Read the model definition and answer for the solid it produces. Units are mm, in the model's axes. A direction names the side the tool comes from. Round coordinates to 2 decimals unless told otherwise and drop trailing zeros. Order: outer loops, then holes, each group sorted by start corner. A loop starts at its lowest first (then second) coordinate and runs counter-clockwise, first axis right, second up.
from build123d import *

# Parameters (mm, degrees)
SKETCH1_R           = 2.286
BOSS_EXTRUDE1_DEPTH = 7.9375
SKETCH2_R           = 2.286
CUT_EXTRUDE1_DEPTH  = 13.335
CUT_EXTRUDE2_START  = 0.79375
CUT_EXTRUDE2_DEPTH  = 2.794
CHAMFER1_SIZE       = 1.5875


with BuildPart() as part:
    # Sketch1 → Boss-Extrude1 (new body)
    with BuildSketch(Plane.XY):
        with BuildLine():
            Line((-5.55625, 4.7625), (-5.55625, 18.0975))
            Line((-5.55625, 18.0975), (5.55625, 18.0975))
            Line((5.55625, 18.0975), (5.55625, 4.7625))
            Line((5.55625, 4.7625), (4.706470588, -0.728382353))
            ThreePointArc((4.706470588, -0.728382353), (0, -4.7625), (-4.706470588, -0.728382353))
            Line((-4.706470588, -0.728382353), (-5.55625, 4.7625))
        make_face()
        with Locations(Location((0, 0, 0), (0, 0, 270))):
            Circle(SKETCH1_R, mode=Mode.SUBTRACT)
    extrude(amount=BOSS_EXTRUDE1_DEPTH)

    # Sketch2 → Cut-Extrude1 (cut)
    with BuildSketch(Plane(origin=(0, 18.0975, 0), x_dir=(1, 0, 0), z_dir=(0, 1, 0))):
        with Locations(Location((2.54e-07, -4.318750409, 0), (0, 0, 270))):
            Circle(SKETCH2_R)
    extrude(amount=-CUT_EXTRUDE1_DEPTH, mode=Mode.SUBTRACT)

    # Sketch3 → Cut-Extrude2 (cut)
    with BuildSketch(Plane(origin=(0, 4.7625, 0), x_dir=(1, 0, 0), z_dir=(0, 1, 0)).offset(CUT_EXTRUDE2_START)):
        Polygon((-1.906410334, -1.016750409), (-4.156524955, -4.914063255), (-4.156524955, -7.9375), (4.156521786, -7.9375), (4.156521786, -4.914056884), (1.906410843, -1.016750409), align=None)
    extrude(amount=CUT_EXTRUDE2_DEPTH, mode=Mode.SUBTRACT)

    # Chamfer1
    chamfer1_edges = [part.edges().sort_by_distance(p)[0] for p in [
        (-5.55625, 18.0975, 3.96875),
        (5.55625, 18.0975, 3.96875),
    ]]
    chamfer(chamfer1_edges, length=CHAMFER1_SIZE)


solid = part.part
Q1. A cutting plane is placed at B-B, the plane y = 8.75. Give the vertices of the cut face in (x, z).
Outcome:
outline: (-5.56, 0) - (5.56, 0) - (5.56, 7.94) - (-5.56, 7.94) - close; hole circle Ø4.57 at (0, 4.32)
Q2. A cutting plane is placed at D-D, the plane y = 0. Give the vertices of the cut face in (x, z), plus the area to 3 significant figures.
Outcome:
outline: (-4.82, 0) - (-2.29, 0) - (-2.29, 7.94) - (-4.82, 7.94) - close; (2.29, 0) - (4.82, 0) - (4.82, 7.94) - (2.29, 7.94) - close
area: 40.2 mm2
Q3. Flat-ended cylindrical pins translate along their axes: pin 1 (4 mm diameter, centred on x = 0, z = 4.32, fed in from +Y); pin 2 (2 mm diameter, centred on x = 1, y = 7, fed in from +Z). Find the tip coordinate at first contact, or state that the pin passes through.
Outcome:
pin 1: stops at y = 4.76
pin 2: stops at z = 1.18
Q4. Straight lines are drawn through the part: probe 1 along X at (y, z) = (10.5, 4.25); probe 2 along Y at (x, z) = (-1.5, 2); probe 3 along X at (y, z) = (6.75, 5.75). For each, find the intervals that lie inside material, in ascending order.
Outcome:
probe 1: x = -5.56 to -2.28, 2.28 to 5.56
probe 2: y = -4.52 to -1.73, 1.73 to 5.56, 8.35 to 18.1
probe 3: x = -5.56 to -4.16, 4.16 to 5.56
Q5. A cutting plane is placed at C-C, the plane z = 5.75. Give the vertices of the cut face in (x, y) (1 decimal).
Outcome:
outline: (-5.6, 4.8) - (-4.7, -0.7) arc R4.8 ccw to (4.7, -0.7) - (5.6, 4.8) - (5.6, 16.5) - (4, 18.1) - (1.8, 18.1) - (1.8, 8.4) - (4.2, 8.4) - (4.2, 5.6) - (1.8, 5.6) - (1.8, 4.8) - (-1.8, 4.8) - (-1.8, 5.6) - (-4.2, 5.6) - (-4.2, 8.4) - (-1.8, 8.4) - (-1.8, 18.1) - (-4, 18.1) - (-5.6, 16.5) - close; hole circle Ø4.6 at (0, 0)
Q6. For a pull along X with two mould halves and no side action, classify faces 1 (the face through (5.556, 11, 4)), 2 (the face through (0.09, -4.76, 3.91)), 3 (the face through (4.157, 7, 6)) as released by +X, released by -X, zero draft, split by the parting line, or undercut.
Outcome:
face 1: released by +X
face 2: split by the parting line
face 3: undercut
Q7. For faces 4 (the face through (1, 18.098, 2)), 5 (the face through (-4.157, 7, 6)), 6 (the face through (-0.88, 13.29, 6.43)), determine the directions among +Z, -Z, +X, -X, +Y, -Y from which every point of the face is accessible in a straight line to the end or side of a thin tool.
Outcome:
face 4: +Z, -Z, +X, -X, +Y
face 5: +Z
face 6: +Y
Q8. A cutting plane is placed at A-A, the plane x = 0. Give the vertices of the cut face in (y, z).
Outcome:
outline: (-4.76, 0) - (-2.29, 0) - (-2.29, 7.94) - (-4.76, 7.94) - close; (2.29, 0) - (18.1, 0) - (18.1, 2.03) - (8.35, 2.03) - (8.35, 1.02) - (5.56, 1.02) - (5.56, 2.03) - (4.76, 2.03) - (4.76, 6.6) - (5.56, 6.6) - (5.56, 7.94) - (2.29, 7.94) - close; (8.35, 6.6) - (18.1, 6.6) - (18.1, 7.94) - (8.35, 7.94) - close
